Print and shaded views of the part. All mm, measured from the part's lowest x, y and z. A direction names the side the tool comes from. Coordinates: 2 decimals unless noted, no trailing zeros. Loops run counter-clockwise (first coordinate to the right, second up) from the corner with the lowest first, then second, coordinate; pieces in that order, holes last.
1) Saw through at C-C, the plane x = 7.25. Write the cut outline in (y, z).
2) Two-plate mould, pull along X, no slides. Class the marked faces 3, 4, 5 and 6: +X half, -X half, draft (parallel to the pull), parting line (faces both ways), or undercut.
3) Saw through at D-D, the plane z = 9.75. Write the cut outline in (x, y).
4) Saw through at A-A, the plane z = 6. Write the cut outline in (x, y) (1 decimal).
5) Which spindle directions (+Z, -Z, +X, -X, +Y, -Y) get a long thin tool onto all of the face, cutting with end or side? Do the marked faces 1 and 2. Say none if no direction does.
6) Wall check: line 1 along Z through (x, y) = (6.5, 3); line 2 along Y through (x, z) = (1.5, 2.75). Give the ranges that are in metal, low to high.
7) Pin check, flat tips, straight feed: pin 1 Ø0.7 at (x, y) = (6, 6.5) entering from -Z; pin 2 Ø1.8 at (x, y) = (6.5, 5.5) entering from +Z; pin 3 Ø4 at (x, z) = (6, 7.5) entering from +Y. Stop position of each tip, or through.
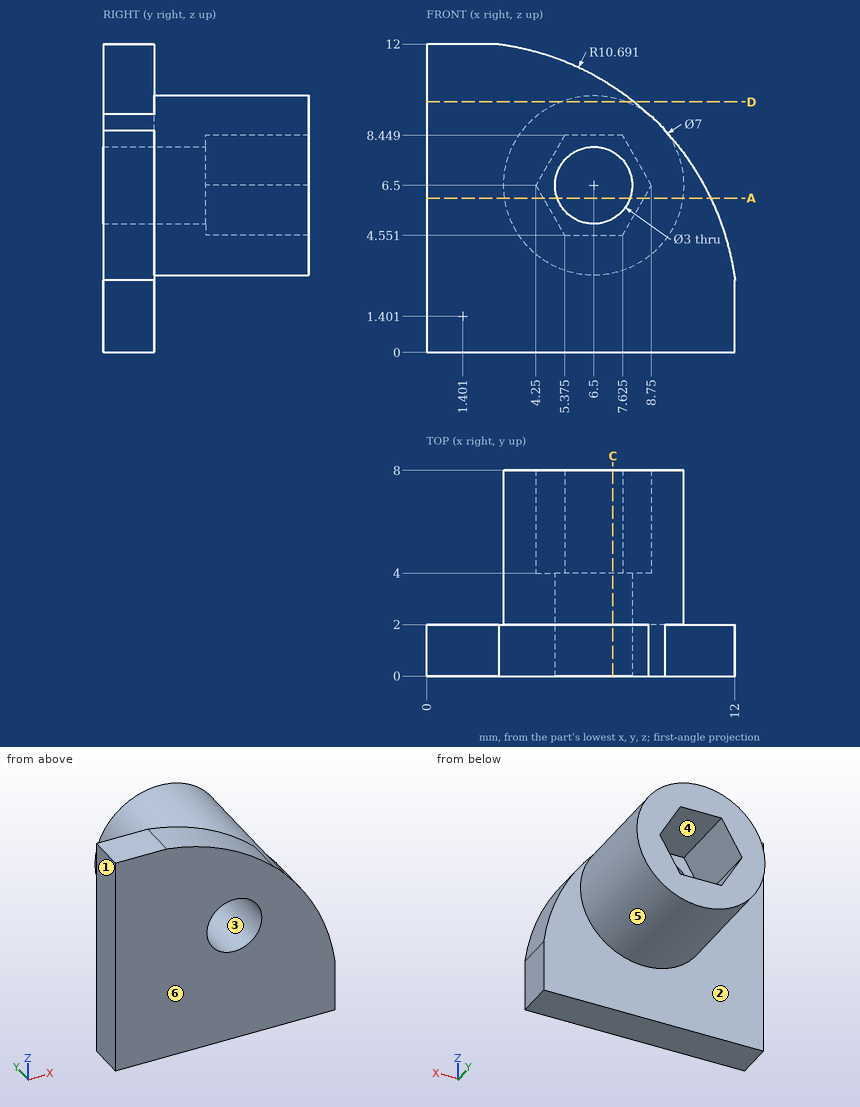
Data:
1. outline: (0, 0) - (2, 0) - (2, 3.08) - (8, 3.08) - (8, 4.55) - (4, 4.55) - (4, 5.2) - (0, 5.2) - close; (0, 7.8) - (4, 7.8) - (4, 8.45) - (8, 8.45) - (8, 9.92) - (2, 9.92) - (2, 10.35) - (0, 10.35) - close
2. face 3: undercut
2. face 4: undercut
2. face 5: parting line
2. face 6: draft
3. outline: (0, 0) - (8.08, 0) - (8.08, 2) - (7.8, 2) - (7.8, 8) - (5.2, 8) - (5.2, 2) - (0, 2) - close
4. outline: (0, 0) - (5.1, 0) - (5.1, 4) - (4.5, 4) - (4.5, 8) - (3, 8) - (3, 2) - (0, 2) - close; (7.9, 0) - (11.1, 0) - (11.1, 2) - (10, 2) - (10, 8) - (8.5, 8) - (8.5, 4) - (7.9, 4) - close
5. face 1: +Z, -Z, -X, +Y, -Y
5. face 2: +Y
6. line 1: z = 3 to 5, 8 to 10
6. line 2: y = 0 to 2
7. pin 1: stops at z = 3
7. pin 2: stops at z = 10
7. pin 3: stops at y = 8
